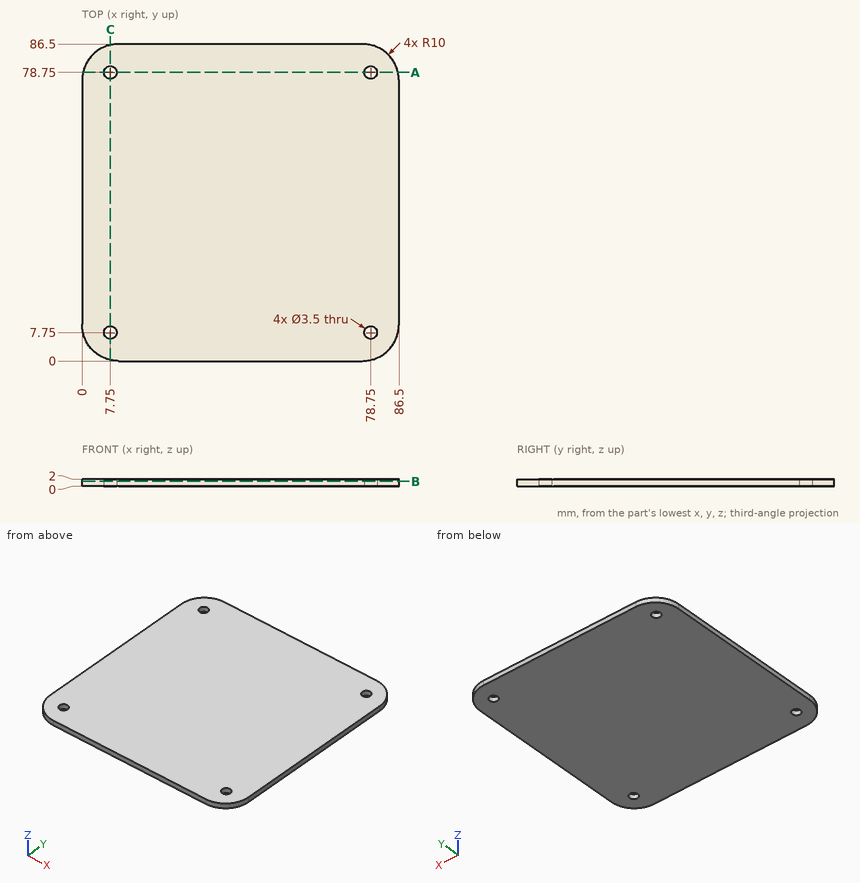
Job drawing, mm, ordinate dimensions from the low corner. One solid piece. Give positions to 0.01 mm unless a question says otherwise; leave off trailing zeros. Loops run counter-clockwise (first coordinate to the right, second up) from the corner with the lowest first, then second, coordinate; pieces in that order, holes last. Notation, with made-up numbers: M 61.5,61 L 84.5,61 A18 cw 84.5,86 Z; hole C 83,2 d5. An arc over 180 degrees is marked long. Return JSON: item names as keys, results as strings.
1) Drill centre lines: line 1 (Y direction, x = 78.75, z = 1.25); line 2 (Y direction, x = 83.5, z = 0.8). Where is each one in solid material? Low to high.
Calculated:
{"line 1": "y = 0.26 to 6, 9.5 to 77, 80.5 to 86.24", "line 2": "y = 2.86 to 83.64"}
2) Saw through at B-B, the plane z = 1.35. List the corners of the cut face in (x, y), then the cut area to 3 significant figures.
Calculated:
{"outline": "M 0,10 A10 ccw 10,0 L 76.5,0 A10 ccw 86.5,10 L 86.5,76.5 A10 ccw 76.5,86.5 L 10,86.5 A10 ccw 0,76.5 Z; hole C 7.75,7.75 d3.5; hole C 7.75,78.75 d3.5; hole C 78.75,7.75 d3.5; hole C 78.75,78.75 d3.5", "area": "7,360 mm2"}
3) Flat gauge pins, fed straight in: pin 1 Ø8 at (x, y) = (20.5, 28.5) entering from -Z; pin 2 Ø2 at (x, y) = (78.75, 7.75) entering from -Z. Where does each tip first touch, or does it go through?
Calculated:
{"pin 1": "stops at z = 0", "pin 2": "passes through"}
4) Saw through at A-A, the plane y = 78.75. List the corners of the cut face in (x, z), then the cut area to 3 significant figures.
Calculated:
{"outline": "M 0.26,0 L 6,0 L 6,2 L 0.26,2 Z; M 9.5,0 L 77,0 L 77,2 L 9.5,2 Z; M 80.5,0 L 86.24,0 L 86.24,2 L 80.5,2 Z", "area": "158 mm2"}
